```python
from build123d import *

# Parameters (mm, degrees)
F1_DEPTH = 25
F2_R     = 7.5
F3_DEPTH = 25
F4_R     = 25
F5_DEPTH = 40


with BuildPart() as f1:
    # F0 (on Top) → F1 (new body)
    with BuildSketch(Plane.XY):
        with BuildLine():
            Line((-17.5, 30.310889), (-47.5, 12.990381))
            ThreePointArc((-47.5, 12.990381), (-55, 0), (-47.5, -12.990381))
            Line((-47.5, -12.990381), (-17.5, -30.310889))
            ThreePointArc((-17.5, -30.310889), (-0.077922, -34.999913), (17.364863, -30.38851))
            Line((17.364863, -30.38851), (47.753373, -13.023647))
            ThreePointArc((47.753373, -13.023647), (55.311289, 0), (47.753373, 13.023647))
            Line((47.753373, 13.023647), (17.364863, 30.38851))
            ThreePointArc((17.364863, 30.38851), (-0.077922, 34.999913), (-17.5, 30.310889))
        make_face()
    extrude(amount=F1_DEPTH)

    # F2 (on face) → F3 (cut)
    with BuildSketch(Plane.XY.offset(25)):
        with Locations((-40, 0)):
            Circle(F2_R)
    extrude(amount=-F3_DEPTH, mode=Mode.SUBTRACT)

    # F4 (on face) → F5 (join)
    with BuildSketch(Plane.XY.offset(25)):
        Circle(F4_R)
    extrude(amount=F5_DEPTH)


solid = f1.part
```
Geometry: final body of the model. Coordinates: model frame, mm. A direction names the side the tool comes from. Give positions to 0.01 mm unless a question says otherwise; leave off trailing zeros. Order: outer loops, then holes, each group sorted by start corner. A loop starts at its lowest first (then second) coordinate and runs counter-clockwise, first axis right, second up. Notation, with made-up numbers: M 25.25,77 L 45.25,77 A10 cw 45.25,86 Z; hole C 84.25,50.25 d9. An arc over 180 degrees is marked long. Answer as CSV lines item,"result". Start each with the question number.
1) Set-up query: faces 4 (the flat face through (0, 0, 65)), 5 (the flat face through (-25, 8, 25)). Return all of +Z, -Z, +X, -X, +Y, -Y with unobstructed straight access to the full face (end or side cutting, diameter ignored); none if empty.
2) Mould query, pull axis Y, two halves, no side actions, for faces 1 (the cylindrical face through (-55, 0, 12)), 2 (the flat face through (-32.71, -21.53, 12.32)), 3 (the cylindrical face through (-32.846, 2.253, 12.675)). Classes: +Y half, -Y half, draft (parallel to the pull), parting line (faces both ways), or undercut.
3) Line query: line 1 (Y direction, x = -40, z = 6.5); line 2 (Z direction, x = 7, y = -25); line 3 (Y direction, x = -46, z = 18). Output: solid intervals per line, ascending. Write a range as from..to.
4) Cut plane C-C (x = -46). Output: boundary loops of the cut face in (y, z), then the cut area to 3 significant figures.
5) Cut plane D-D (y = 9). Output: boundary loops of the cut face in (x, z), then the cut area to 3 significant figures.
6) First-contact query: P1, Ø3, axis at y = -9, z = 10.5, coming from the +X side; P2, Ø5, axis at x = 15.5, y = 26.5, coming from the +Z side; P3, Ø1, axis at x = -41, z = 23, coming from the -Y side; P4, Ø4, axis at x = 28, y = -14.5, coming from the -Z side. Flat tips, straight axial feed; report the tip coordinate or a pass-through.
7) Cut plane A-A (y = 0). Output: boundary loops of the cut face in (x, z), then the cut area to 3 significant figures.
8) Cut plane B-B (x = 0). Output: boundary loops of the cut face in (y, z).
Findings below:
1,face 4,"+Z, +X, -X, +Y, -Y"
1,face 5,"+Z"
2,face 1,"parting line"
2,face 2,"-Y half"
2,face 3,"undercut"
3,line 1,"y = -17.32..-7.5, 7.5..17.32"
3,line 2,"z = 0..25"
3,line 3,"y = -13.86..-4.5, 4.5..13.86"
4,outline,"M -13.86,0 L -4.5,0 L -4.5,25 L -13.86,25 Z; M 4.5,0 L 13.86,0 L 13.86,25 L 4.5,25 Z"
4,area,"468 mm²"
5,outline,"M -52,0 L 52.31,0 L 52.31,25 L 23.32,25 L 23.32,65 L -23.32,65 L -23.32,25 L -52,25 Z"
5,area,"4,470 mm²"
6,P1,"stops at x = 53.3"
6,P2,"stops at z = 25"
6,P3,"stops at y = -17.03"
6,P4,"stops at z = 0"
7,outline,"M -55,0 L -47.5,0 L -47.5,25 L -55,25 Z; M -32.5,0 L 55.31,0 L 55.31,25 L 25,25 L 25,65 L -25,65 L -25,25 L -32.5,25 Z"
7,area,"4,380 mm²"
8,outline,"M -35,0 L 35,0 L 35,25 L 25,25 L 25,65 L -25,65 L -25,25 L -35,25 Z"
